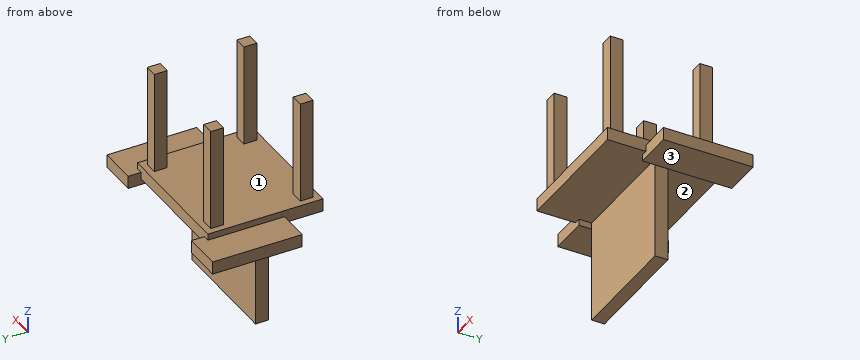
```python
from build123d import *

# Parameters (mm, degrees)
SKETCH_1_W      = 500
SKETCH_1_H      = 450
EXTRUDE_1_DEPTH = 50
SKETCH_2_W      = 50
SKETCH_2_H      = 50
EXTRUDE_2_DEPTH = 450
SKETCH_3_W      = 50
SKETCH_3_H      = 50
EXTRUDE_3_DEPTH = 450
SKETCH_4_W      = 50
SKETCH_4_H      = 50
EXTRUDE_4_DEPTH = 450
SKETCH_5_W      = 50
SKETCH_5_H      = 50
EXTRUDE_5_DEPTH = 450
SKETCH_6_W      = 450
SKETCH_6_H      = 50
EXTRUDE_6_DEPTH = 400
SKETCH_7_W      = 50
SKETCH_7_H      = 350
EXTRUDE_7_DEPTH = 150
SKETCH_8_W      = 50
SKETCH_8_H      = 350
EXTRUDE_8_DEPTH = 150


with BuildPart() as part:
    # 草图1 → 凸台-拉伸1 (new body)
    with BuildSketch(Plane.XY):
        Rectangle(SKETCH_1_W, SKETCH_1_H)
    extrude(amount=EXTRUDE_1_DEPTH)

    # 草图2 → 凸台-拉伸2 (add)
    with BuildSketch(Plane.XY):
        with Locations((-200, -175)):
            Rectangle(SKETCH_2_W, SKETCH_2_H)
    extrude(amount=EXTRUDE_2_DEPTH)

    # 草图3 → 凸台-拉伸3 (add)
    with BuildSketch(Plane.XY):
        with Locations((200, -175)):
            Rectangle(SKETCH_3_W, SKETCH_3_H)
    extrude(amount=EXTRUDE_3_DEPTH)

    # 草图4 → 凸台-拉伸4 (add)
    with BuildSketch(Plane.XY):
        with Locations((-200, 175)):
            Rectangle(SKETCH_4_W, SKETCH_4_H)
    extrude(amount=EXTRUDE_4_DEPTH)

    # 草图5 → 凸台-拉伸5 (add)
    with BuildSketch(Plane.XY):
        with Locations((200, 175)):
            Rectangle(SKETCH_5_W, SKETCH_5_H)
    extrude(amount=EXTRUDE_5_DEPTH)

    # 草图6 → 凸台-拉伸6 (add)
    with BuildSketch(Plane(origin=(0, 0, 0), x_dir=(-1, 0, 0), z_dir=(0, 0, -1))):
        Rectangle(SKETCH_6_W, SKETCH_6_H)
    extrude(amount=EXTRUDE_6_DEPTH)

    # 草图7 → 凸台-拉伸7 (add)
    with BuildSketch(Plane.ZY.offset(225)):
        with Locations((0, 100)):
            Rectangle(SKETCH_7_W, SKETCH_7_H)
    extrude(amount=EXTRUDE_7_DEPTH)

    # 草图8 → 凸台-拉伸8 (add)
    with BuildSketch(Plane(origin=(225, 0, 0), x_dir=(0, 0, -1), z_dir=(1, 0, 0))):
        with Locations((0, 100)):
            Rectangle(SKETCH_8_W, SKETCH_8_H)
    extrude(amount=EXTRUDE_8_DEPTH)


solid = part.part
```
CAD build for the part. Positions are in the model's coordinates, mm. Face numbers are marked on the shaded views. Give positions to 0.01 mm unless a question says otherwise; leave off trailing zeros. Loops run counter-clockwise (first coordinate to the right, second up) from the corner with the lowest first, then second, coordinate; pieces in that order, holes last. Notation, with made-up numbers: (87, 59.25) -> (144, 59.25) arc R27 ccw to (144, 98.25) -> close; hole circle Ø2 at (-26, 7). An arc over 180 degrees is marked (long way). Use a Markdown table: item, result.
1. Flat gauge pins, fed straight in: pin 1 (15 mm diameter, centred on y = 183, z = 295, fed in from +X); pin 2 (25 mm diameter, centred on x = -190, z = 208.5, fed in from +Y); pin 3 (5 mm diameter, centred on x = -43, y = -55.5, fed in from +Z). Where does each tip first touch, or does it go through?
Check result:
| item | result |
|---|---|
| pin 1 | stops at x = 225 |
| pin 2 | stops at y = 200 |
| pin 3 | stops at z = 50 |
2. Slice it at D-D (y = -173.5). List the corners of the cut face in (x, z), plus the area to 3 significant figures.
Check result:
| item | result |
|---|---|
| outline | (-250, 0) -> (250, 0) -> (250, 50) -> (225, 50) -> (225, 450) -> (175, 450) -> (175, 50) -> (-175, 50) -> (-175, 450) -> (-225, 450) -> (-225, 50) -> (-250, 50) -> close |
| area | 65,000 mm^2 |
3. Wall check: L1, parallel to X at y = -176.5, z = 353; L2, parallel to Y at x = -181.5, z = 36; L3, parallel to Z at x = 258, y = 121.5. Give the ranges that are in metal, low to high. Write a range as [from, to].
Check result:
| item | result |
|---|---|
| L1 | x = [-225, -175], [175, 225] |
| L2 | y = [-225, 225] |
| L3 | z = [-25, 25] |
4. Slice it at C-C (x = 104). List the corners of the cut face in (y, z), plus the area to 3 significant figures.
Check result:
| item | result |
|---|---|
| outline | (-225, 0) -> (-25, 0) -> (-25, -400) -> (25, -400) -> (25, 0) -> (225, 0) -> (225, 50) -> (-225, 50) -> close |
| area | 42,500 mm^2 |
5. Mould opens along X. For the marked faces 1, 2 and 3 say: pulls with the +X half, pulls with the -X half, needs draft (parallel to the pull), parting line crosses it, or undercut.
Check result:
| item | result |
|---|---|
| face 1 | undercut |
| face 2 | undercut |
| face 3 | needs draft |
6. Slice it at B-B (y = 84). List the corners of the cut face in (x, z).
Check result:
| item | result |
|---|---|
| outline | (-375, -25) -> (-225, -25) -> (-225, 0) -> (225, 0) -> (225, -25) -> (375, -25) -> (375, 25) -> (250, 25) -> (250, 50) -> (-250, 50) -> (-250, 25) -> (-375, 25) -> close |
7. Slice it at A-A (z = 273). List the corners of the cut face in (x, y).
Check result:
| item | result |
|---|---|
| outline | (-225, -200) -> (-175, -200) -> (-175, -150) -> (-225, -150) -> close; (-225, 150) -> (-175, 150) -> (-175, 200) -> (-225, 200) -> close; (175, -200) -> (225, -200) -> (225, -150) -> (175, -150) -> close; (175, 150) -> (225, 150) -> (225, 200) -> (175, 200) -> close |
